```python
from build123d import *

# Parameters (mm, degrees)
EXTRUDE_1_DEPTH          = 4
CUT_EXTRUDE_1_DEPTH      = 2
CUT_EXTRUDE_1_DEPTH_BACK = 2
CUT_EXTRUDE_2_DEPTH      = 9


with BuildPart() as part:
    # 草图1 → 凸台-拉伸1 (new body, symmetric)
    with BuildSketch(Plane.XY):
        with BuildLine():
            Line((-92.895446795, 4.408623913), (-106.879707603, 5.072287728))
            ThreePointArc((-106.879707603, 5.072287728), (-106.030919043, 14.368166442), (-104.375171166, 23.554694734))
            Line((-104.375171166, 23.554694734), (-90.718606715, 20.472772059))
            ThreePointArc((-90.718606715, 20.472772059), (-92.157714682, 12.488219431), (-92.895446795, 4.408623913))
        make_face()
    extrude(amount=EXTRUDE_1_DEPTH, both=True)

    # 草图2 → 切除-拉伸1 (cut, two sides)
    with BuildSketch(Plane.XY) as cut_extrude_1_sk:
        with BuildLine():
            Line((-104.881956059, 4.977478611), (-106.879707603, 5.072287728))
            ThreePointArc((-106.879707603, 5.072287728), (-106.030919043, 14.368166442), (-104.375171166, 23.554694734))
            Line((-104.375171166, 23.554694734), (-102.424233387, 23.114420066))
            ThreePointArc((-102.424233387, 23.114420066), (-104.049032706, 14.099602583), (-104.881956059, 4.977478611))
        make_face()
        with BuildLine():
            Line((-80.070774139, 18.069839991), (-92.669544493, 20.913046727))
            ThreePointArc((-92.669544493, 20.913046727), (-94.139601019, 12.75678329), (-94.893198339, 4.503433029))
            Line((-94.893198339, 4.503433029), (-81.992113947, 3.891174505))
            ThreePointArc((-81.992113947, 3.891174505), (-81.340970995, 11.022451002), (-80.070774139, 18.069839991))
        make_face()
    extrude(amount=CUT_EXTRUDE_1_DEPTH, mode=Mode.SUBTRACT)
    extrude(cut_extrude_1_sk.sketch, amount=-CUT_EXTRUDE_1_DEPTH_BACK, mode=Mode.SUBTRACT)

    # 草图3 → 切除-拉伸2 (cut, through all)
    with BuildSketch(Plane.XY.offset(4)):
        with BuildLine():
            ThreePointArc((-96.785643699, 14.691278047), (-97.964954769, 15.293433182), (-99.261988484, 15.026845581))
            Line((-99.261988484, 15.026845581), (-98.233518627, 13.311546845))
            Line((-98.233518627, 13.311546845), (-96.785643699, 14.691278047))
        make_face()
        with BuildLine():
            Line((-98.233518627, 13.311546845), (-99.261988484, 15.026845581))
            ThreePointArc((-99.261988484, 15.026845581), (-100.215404965, 13.580110704), (-99.681393556, 11.931815643))
            Line((-99.681393556, 11.931815643), (-98.233518627, 13.311546845))
        make_face()
        with BuildLine():
            Line((-96.785643699, 14.691278047), (-98.233518627, 13.311546845))
            Line((-98.233518627, 13.311546845), (-97.205048771, 11.596248109))
            ThreePointArc((-97.205048771, 11.596248109), (-96.493268687, 12.325884558), (-96.233518627, 13.311546845))
            ThreePointArc((-96.233518627, 13.311546845), (-96.376673203, 14.054598035), (-96.785643699, 14.691278047))
        make_face()
        with BuildLine():
            Line((-97.205048771, 11.596248109), (-98.233518627, 13.311546845))
            Line((-98.233518627, 13.311546845), (-99.681393556, 11.931815643))
            ThreePointArc((-99.681393556, 11.931815643), (-98.502082486, 11.329660508), (-97.205048771, 11.596248109))
        make_face()
    extrude(amount=-CUT_EXTRUDE_2_DEPTH, mode=Mode.SUBTRACT)


solid = part.part
```
Geometry check sheet. Reference: the model listing, model coordinates, mm. A direction names the side the tool comes from. Coordinates: 2 decimals unless noted, no trailing zeros. Write each loop counter-clockwise with the first axis right and the second up, starting at its lowest first coordinate (ties: lowest second). Pieces come first, ordered by that corner, then holes. Notation, with made-up numbers: (53.25, -27.75) -> (102.25, -27.75) arc R20 cw to (102.25, 6.25) -> close; hole circle Ø1 at (79, -35). An arc over 180 degrees is marked (long way). Use CSV: the item, a comma, the result in double quotes. Start each with the question number.
Item 1: Thickness scan on line 1 (Z direction, x = -92.5, y = 12); line 2 (X direction, y = 13, z = 1); line 3 (Y direction, x = -97.25, z = -3). Record the ranges inside material, lowest first.
Item 2: Depth check by flat-ended pin: pin 1 Ø3 at (x, z) = (-103, 2.5) entering from -Y; pin 2 Ø1.5 at (y, z) = (13.5, 2.5) entering from -X; pin 3 Ø1.5 at (x, z) = (-103.5, 3) entering from +Y. Enter the tip coordinate at first touch or a pass-through.
Item 3: Cross-section at C-C, the plane y = 21.5. Record the cut outline in (x, z).
Item 4: Cross-section at A-A, the plane z = 3. Record the cut outline in (x, y).
Item 5: Cross-section at D-D, the plane x = -93.75. Record the cut outline in (y, z).
Item 6: Mould release check, pull along Z, two halves, no side actions. Record for faces 4 (the flat face through (-97.642, 22.035, 0.056)), 5 (the flat face through (-100.5, 14.1, -4)), 6 (the flat face through (-93, 13, 2)): released by +Z, released by -Z, zero draft, split by the parting line, or undercut.
Item 7: Cross-section at B-B, the plane x = -98.5. Record the cut outline in (y, z), plus the area to 3 significant figures.
Item 8: Set-up check for faces 1 (the flat face through (-105, 14, 2)), 2 (the cylindrical face through (-94.124, 12.872, 0.028)), 3 (the cylindrical face through (-106.05, 14.24, 3.01)): record each of +Z, -Z, +X, -X, +Y, -Y from which the full face is reachable in a straight line by a thin tool's end or side.
Answers:
1,line 1,"-4 to -2, 2 to 4"
1,line 2,"-104.19 to -100.21, -96.26 to -94.11"
1,line 3,"4.62 to 11.57, 15.05 to 21.95"
2,pin 1,"y = 4.82"
2,pin 2,"x = -106.24"
2,pin 3,"y = 23.53"
3,outline,"(-104.82, -4) -> (-95.27, -4) -> (-95.27, 4) -> (-104.82, 4) -> (-104.82, 2) -> (-102.78, 2) -> (-102.78, -2) -> (-104.82, -2) -> close"
4,outline,"(-106.88, 5.07) -> (-92.9, 4.41) arc R93 cw to (-90.72, 20.47) -> (-104.38, 23.55) arc R107 ccw to start; hole circle Ø4 at (-98.23, 13.31)"
5,outline,"(4.45, -4) -> (21.16, -4) -> (21.16, 4) -> (4.45, 4) -> (4.45, 2) -> (15.36, 2) -> (15.36, -2) -> (4.45, -2) -> close"
6,face 4,"zero draft"
6,face 5,"released by -Z"
6,face 6,"undercut"
7,outline,"(4.67, -4) -> (11.33, -4) -> (11.33, 4) -> (4.67, 4) -> close; (15.29, -4) -> (22.23, -4) -> (22.23, 4) -> (15.29, 4) -> close"
7,area,"109 mm^2"
8,face 1,"-X, +Y"
8,face 2,"+X, -Y"
8,face 3,"+Z, -Z, -X, +Y"
